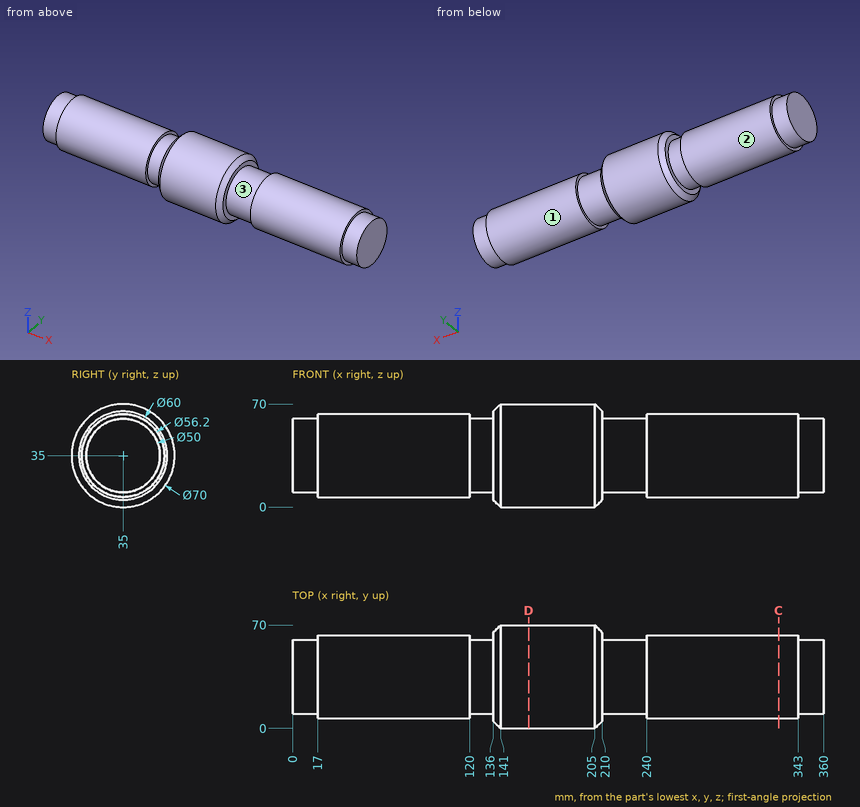
Input: dimensioned drawing with shaded views. Units: mm. Origin: part minimum x, y, z. A direction names the side the tool comes from. Round coordinates to 2 decimals unless told otherwise and drop trailing zeros. Order: outer loops, then holes, each group sorted by start corner. A loop starts at its lowest first (then second) coordinate and runs counter-clockwise, first axis right, second up. Notation, with made-up numbers: (26.25, 87.5) -> (39.25, 87.5) arc R17 ccw to (39.25, 99.5) -> close; hole circle Ø7 at (-7, 83.25). An arc over 180 degrees is marked (long way). Put each result on its own line as item: value. Start each with the question number.
Q1. First-contact query: pin 1 (8 mm diameter, centred on x = 155.5, z = 46, fed in from -Y); pin 2 (1 mm diameter, centred on y = 57, z = 60.5, fed in from -X); pin 3 (8 mm diameter, centred on x = 280, z = 19.5, fed in from -Y); pin 4 (18 mm diameter, centred on y = 29, z = 45.5, fed in from -X). Flat tips, straight axial feed; report the tip coordinate or a pass-through.
Q2. Section C-C on x = 329.5. Return the cut outline in (y, z).
Q3. Line query: probe 1 along X at (y, z) = (46, 11); probe 2 along Y at (x, z) = (140, 51); probe 3 along Z at (x, y) = (144, 33). Output: solid intervals per line, ascending.
Q4. Section D-D on x = 160. Return the cut outline in (y, z).
Q5. Reachability of the marked faces 1, 2 and 3 from +Z, -Z, +X, -X, +Y, -Y: full face, straight path, thin tool, end or side. Return the list, or none.
Ans:
1. pin 1: stops at y = 0.71
1. pin 2: stops at x = 139.18
1. pin 3: stops at y = 9.36
1. pin 4: stops at x = 0
2. outline: circle Ø56.2 at (35, 35)
3. probe 1: x = 17 to 120, 136 to 210, 240 to 343
3. probe 2: y = 5 to 65
3. probe 3: z = 0.06 to 69.94
4. outline: circle Ø70 at (35, 35)
5. face 1: +X
5. face 2: -X
5. face 3: none
